Geometry: final body of the model. Coordinates: model frame, mm. A direction names the side the tool comes from. Round coordinates to 2 decimals unless told otherwise and drop trailing zeros. Write each loop counter-clockwise with the first axis right and the second up, starting at its lowest first coordinate (ties: lowest second). Pieces come first, ordered by that corner, then holes. Notation, with made-up numbers: M 23,39.25 L 79,39.25 A28 cw 79,63.25 Z; hole C 68.25,89.5 d2. An arc over 180 degrees is marked long. Use one line per item in the form item = value. Start each with the question number.
Item 1: Pin query (flat end, axial travel): pin 1 Ø3 at (y, z) = (0, 4.75) entering from -X; pin 2 Ø1 at (x, y) = (2.5, -9) entering from +Z; pin 3 Ø1.2 at (x, z) = (2, 27.5) entering from -Y. Return the tip coordinate at first contact, or that it passes through.
Item 2: Section query B-B (y = 0). Return loops of the section in (x, z) (3 decimals), and give its area (3 significant figures).
Item 3: Ray query, probe 1 along Y at (x, z) = (2.5, -4.75) (3 decimals); probe 2 along Y at (x, z) = (2.5, -30); probe 3 along Z at (x, y) = (0.3, -0.5). Return the intervals inside material, ascending.
Item 4: Section query D-D (z = -4.75). Return loops of the section in (x, y) (3 decimals).
Item 5: Section query A-A (z = 30). Return loops of the section in (x, y), and give its area (3 significant figures).
Item 6: Reachability of faces 1 (the cylindrical face through (2.03, -11.99, -42.15)), 2 (the flat face through (2, -5, 29)) from +Z, -Z, +X, -X, +Y, -Y: full face, straight path, thin tool, end or side. Return the list, or none.
Item 7: Section query C-C (x = 2.3). State how many separate pieces and enclosed holes the cut face has, and give its area (3 significant figures).
Item 8: Pull-direction query (Y, two-part tool) for faces 3 (the cylindrical face through (1.97, -1.99, 42.15)), 4 (the cylindrical face through (2.028, -0.479, 28.845)), 5 (the flat face through (0, 0, -1)), 6 (the cylindrical face through (2.03, 12.15, -41.99)); classes: pulls with the +Y half, pulls with the -Y half, needs draft (parallel to the pull), parting line crosses it, or undercut.
from build123d import *

# Parameters (mm, degrees)
SKETCH1_W           = 90
SKETCH1_H           = 30
BOSS_EXTRUDE1_DEPTH = 4
SKETCH6_R           = 1.575
CUT_EXTRUDE6_DEPTH  = 48.602520942
SKETCH7_R           = 1.575
CUT_EXTRUDE7_DEPTH  = 48.602520942
SKETCH13_R          = 1.25
CUT_EXTRUDE13_DEPTH = 48.602520942
SKETCH14_R          = 1.25
CUT_EXTRUDE14_DEPTH = 48.602520942
SKETCH15_W          = 15
SKETCH15_H          = 10
CUT_EXTRUDE15_DEPTH = 48.602520942
FILLET1_R           = 10
SKETCH16_W          = 20
SKETCH16_H          = 10
CUT_EXTRUDE16_DEPTH = 48.602520942
FILLET2_R           = 10
BOSS_EXTRUDE2_DEPTH = 4
FILLET3_R           = 10


with BuildPart() as part:
    # Sketch1 → Boss-Extrude1 (new body)
    with BuildSketch(Plane(origin=(0, 0, 0), x_dir=(0, 0, -1), z_dir=(1, 0, 0))):
        Rectangle(SKETCH1_W, SKETCH1_H)
    extrude(amount=BOSS_EXTRUDE1_DEPTH)

    # Sketch6 → Cut-Extrude6 (cut, through all)
    with BuildSketch(Plane(origin=(4, 0, 0), x_dir=(0, 0, -1), z_dir=(1, 0, 0))):
        with Locations((-4.75, 0)):
            Circle(SKETCH6_R)
    extrude(amount=-CUT_EXTRUDE6_DEPTH, mode=Mode.SUBTRACT)

    # Sketch7 → Cut-Extrude7 (cut, through all)
    with BuildSketch(Plane(origin=(4, 0, 0), x_dir=(0, 0, -1), z_dir=(1, 0, 0))):
        with Locations((4.75, 0)):
            Circle(SKETCH7_R)
    extrude(amount=-CUT_EXTRUDE7_DEPTH, mode=Mode.SUBTRACT)

    # Sketch13 → Cut-Extrude13 (cut, through all)
    with BuildSketch(Plane(origin=(4, 0, 0), x_dir=(0, 0, -1), z_dir=(1, 0, 0))):
        with Locations((-30, 0)):
            Circle(SKETCH13_R)
    extrude(amount=-CUT_EXTRUDE13_DEPTH, mode=Mode.SUBTRACT)

    # Sketch14 → Cut-Extrude14 (cut, through all)
    with BuildSketch(Plane(origin=(4, 0, 0), x_dir=(0, 0, -1), z_dir=(1, 0, 0))):
        with Locations((30, 0)):
            Circle(SKETCH14_R)
    extrude(amount=-CUT_EXTRUDE14_DEPTH, mode=Mode.SUBTRACT)

    # Sketch15 → Cut-Extrude15 (cut, through all)
    with BuildSketch(Plane(origin=(4, 0, 0), x_dir=(0, 0, -1), z_dir=(1, 0, 0))):
        with Locations((-37.5, -10)):
            Rectangle(SKETCH15_W, SKETCH15_H)
    extrude(amount=-CUT_EXTRUDE15_DEPTH, mode=Mode.SUBTRACT)

    # Fillet1
    fillet1_edges = [part.edges().sort_by_distance(p)[0] for p in [
        (2, -15, -45),
        (2, 15, 45),
        (2, 15, -45),
    ]]
    fillet(fillet1_edges, radius=FILLET1_R)

    # Sketch16 → Cut-Extrude16 (cut, through all)
    with BuildSketch(Plane(origin=(4, 0, 0), x_dir=(0, 0, -1), z_dir=(1, 0, 0))):
        with Locations((-20, -10)):
            Rectangle(SKETCH16_W, SKETCH16_H)
    extrude(amount=-CUT_EXTRUDE16_DEPTH, mode=Mode.SUBTRACT)

    # Fillet2
    fillet2_edges = [part.edges().sort_by_distance(p)[0] for p in [
        (2, -5, 45),
    ]]
    fillet(fillet2_edges, radius=FILLET2_R - 0.0001)  # a hair under: the kernel refuses the full size

    # Sketch17 → Boss-Extrude2 (add)
    with BuildSketch(Plane(origin=(4, 0, 0), x_dir=(0, 0, -1), z_dir=(1, 0, 0))):
        with BuildLine():
            Line((-22.5, -5), (-10, -5))
            Line((-10, -5), (-10, -15))
            add(Edge.make_bspline(
                [(-10, -15), (-10.926575713, -9.745128006), (-15.532860799, -6.228494619), (-22.5, -5)],
                knots=[0, 0, 0, 0, 1, 1, 1, 1], degree=3))
        make_face()
    extrude(amount=-BOSS_EXTRUDE2_DEPTH)

    # Fillet3
    fillet3_edges = [part.edges().sort_by_distance(p)[0] for p in [
        (2, -15, 10),
    ]]
    fillet(fillet3_edges, radius=FILLET3_R)


solid = part.part
Working result:
q1.pin_1 = through
q1.pin_2 = 13.97
q1.pin_3 = -5
q2.outline = M 0,-45 L 4,-45 L 4,-31.25 L 0,-31.25 Z; M 0,-28.75 L 4,-28.75 L 4,-6.325 L 0,-6.325 Z; M 0,-3.175 L 4,-3.175 L 4,3.175 L 0,3.175 Z; M 0,6.325 L 4,6.325 L 4,28.75 L 0,28.75 Z; M 0,31.25 L 4,31.25 L 4,43.66 L 0,43.66 Z
q2.area = 309 mm²
q3.probe_1 = -15 to -1.575, 1.575 to 15
q3.probe_2 = -15 to -1.25, 1.25 to 15
q3.probe_3 = -45 to -31.15, -28.85 to -6.24, -3.26 to 3.26, 6.24 to 28.85, 31.15 to 43.35
q4.outline = M 0,-15 L 4,-15 L 4,-1.575 L 0,-1.575 Z; M 0,1.575 L 4,1.575 L 4,15 L 0,15 Z
q5.outline = M 0,-5 L 4,-5 L 4,-1.25 L 0,-1.25 Z; M 0,1.25 L 4,1.25 L 4,15 L 0,15 Z
q5.area = 70.0 mm²
q6.face_1 = -Z, +X, -X, -Y
q6.face_2 = +Z, +X, -X, -Y
q7.separate_pieces = 1
q7.enclosed_holes = 4
q7.area = 2,270 mm²
q8.face_3 = pulls with the -Y half
q8.face_4 = undercut
q8.face_5 = needs draft
q8.face_6 = pulls with the +Y half
